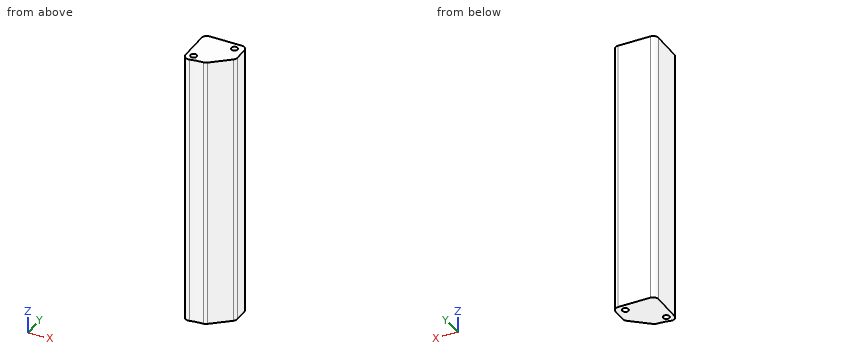
```python
from build123d import *

# Parameters (mm, degrees)
BOSS_EXTRUDE1_DEPTH                    = 77.66
M2_2X0_45_TAPPED_HOLE1_D               = 1.75
M2_2X0_45_TAPPED_HOLE1_DEPTH           = 10
M2_2X0_45_TAPPED_HOLE1_TIP             = 0.525753042
M2_2X0_45_TAPPED_HOLE1_ON_FACE_2_D     = 1.75
M2_2X0_45_TAPPED_HOLE1_ON_FACE_2_DEPTH = 10
M2_2X0_45_TAPPED_HOLE1_ON_FACE_2_TIP   = 0.525753042
FILLET1_R                              = 1.5


with BuildPart() as part:
    # Sketch1 → Boss-Extrude1 (new body)
    with BuildSketch(Plane.XY):
        with BuildLine():
            Line((0, 0), (0, 12))
            Line((0, 12), (12, 12))
            Line((12, 12), (12, 6))
            Line((12, 6), (6, 0.998499343))
            ThreePointArc((6, 0.998499343), (2.961819318, 0.728678054), (0, 0))
        make_face()
    extrude(amount=BOSS_EXTRUDE1_DEPTH)

    # M2.2x0.45 Tapped Hole1
    with Locations(Plane(origin=(2, 2.5, 77.66), x_dir=(1, 0, 0), z_dir=(0, 0, 1))):
        with Locations((0, 0), (7.5, 7.5)):
            Hole(M2_2X0_45_TAPPED_HOLE1_D / 2, depth=M2_2X0_45_TAPPED_HOLE1_DEPTH)
            with Locations((0, 0, -(M2_2X0_45_TAPPED_HOLE1_DEPTH + M2_2X0_45_TAPPED_HOLE1_TIP / 2))):  # 118° drill point
                Cone(0, M2_2X0_45_TAPPED_HOLE1_D / 2, M2_2X0_45_TAPPED_HOLE1_TIP, mode=Mode.SUBTRACT)

    # M2.2x0.45 Tapped Hole1 on face 2
    with Locations(Plane(origin=(2, 2.5, 0), x_dir=(-1, 0, 0), z_dir=(0, 0, -1))):
        with Locations((0, 0), (-7.5, 7.5)):
            Hole(M2_2X0_45_TAPPED_HOLE1_ON_FACE_2_D / 2, depth=M2_2X0_45_TAPPED_HOLE1_ON_FACE_2_DEPTH)
            with Locations((0, 0, -(M2_2X0_45_TAPPED_HOLE1_ON_FACE_2_DEPTH + M2_2X0_45_TAPPED_HOLE1_ON_FACE_2_TIP / 2))):  # 118° drill point
                Cone(0, M2_2X0_45_TAPPED_HOLE1_ON_FACE_2_D / 2, M2_2X0_45_TAPPED_HOLE1_ON_FACE_2_TIP, mode=Mode.SUBTRACT)

    # Fillet1
    fillet1_edges = [part.edges().sort_by_distance(p)[0] for p in [
        (0, 0, 38.83),
        (0, 12, 38.83),
        (12, 12, 38.83),
        (12, 6, 38.83),
        (6, 0.998499343, 38.83),
    ]]
    fillet(fillet1_edges, radius=FILLET1_R)


solid = part.part
```
Read the model definition and answer for the solid it produces. Units are mm, in the model's axes. Coordinates: 2 decimals unless noted, no trailing zeros. Loops run counter-clockwise (first coordinate to the right, second up) from the corner with the lowest first, then second, coordinate; pieces in that order, holes last. Notation, with made-up numbers: (-30, -6.75) -> (-19, -6.75) arc R22 ccw to (-19, 30.25) -> close; hole circle Ø8 at (-20.75, -12.75). An arc over 180 degrees is marked (long way). Return JSON: item names as keys, results as strings.
Item 1: Find section C-C (y = 4.75). Determine the outline of the cut face in (x, z), plus the area to 3 significant figures.
Answers:
{"outline": "(0, 0) -> (10.5, 0) -> (10.5, 77.66) -> (0, 77.66) -> close", "area": "815 mm2"}
Item 2: Find section A-A (z = 55.5). Determine the outline of the cut face in (x, y) (3 decimals), plus the area to 3 significant figures.
Answers:
{"outline": "(0, 1.97) arc R1.5 ccw to (1.831, 0.507) arc R20 cw to (5.497, 0.986) arc R1.5 ccw to (6.401, 1.333) -> (11.46, 5.55) arc R1.5 ccw to (12, 6.702) -> (12, 10.5) arc R1.5 ccw to (10.5, 12) -> (1.5, 12) arc R1.5 ccw to (0, 10.5) -> close", "area": "117 mm2"}
Item 3: Find section B-B (x = 4.75). Determine the outline of the cut face in (y, z), plus the area to 3 significant figures.
Answers:
{"outline": "(0.94, 0) -> (12, 0) -> (12, 77.66) -> (0.94, 77.66) -> close", "area": "859 mm2"}
Item 4: Flat-ended cylindrical pins translate along their axes: P1, Ø1.4, axis at x = 2, y = 2.5, coming from the -Z side; P2, Ø1.6, axis at x = 9.5, y = 10, coming from the -Z side; P3, Ø1.6, axis at x = 2, y = 2.5, coming from the +Z side. Find the tip coordinate at first contact, or state that the pin passes through.
Answers:
{"P1": "stops at z = 10.11", "P2": "stops at z = 10.05", "P3": "stops at z = 67.61"}
Item 5: Find the intervals of material crossed by probe 1 along X at (y, z) = (10, 69.5) (3 decimals); probe 2 along Y at (x, z) = (7, 18); probe 3 along Y at (x, z) = (8.25, 39), in increasing order.
Answers:
{"probe 1": "x = 0 to 8.625, 10.375 to 12", "probe 2": "y = 1.83 to 12", "probe 3": "y = 2.87 to 12"}
